Could you check a few things on this drawing? It's one solid part, dimensions in mm from its lowest x, y, z. A direction names the side the tool comes from. Round coordinates to 2 decimals unless told otherwise and drop trailing zeros. Write each loop counter-clockwise with the first axis right and the second up, starting at its lowest first coordinate (ties: lowest second). Pieces come first, ordered by that corner, then holes. Notation, with made-up numbers: (45, 86) -> (61, 86) arc R21 ccw to (61, 96) -> close; hole circle Ø3 at (16, 88.25). An arc over 180 degrees is marked (long way). Answer in a Markdown table with one row per item.
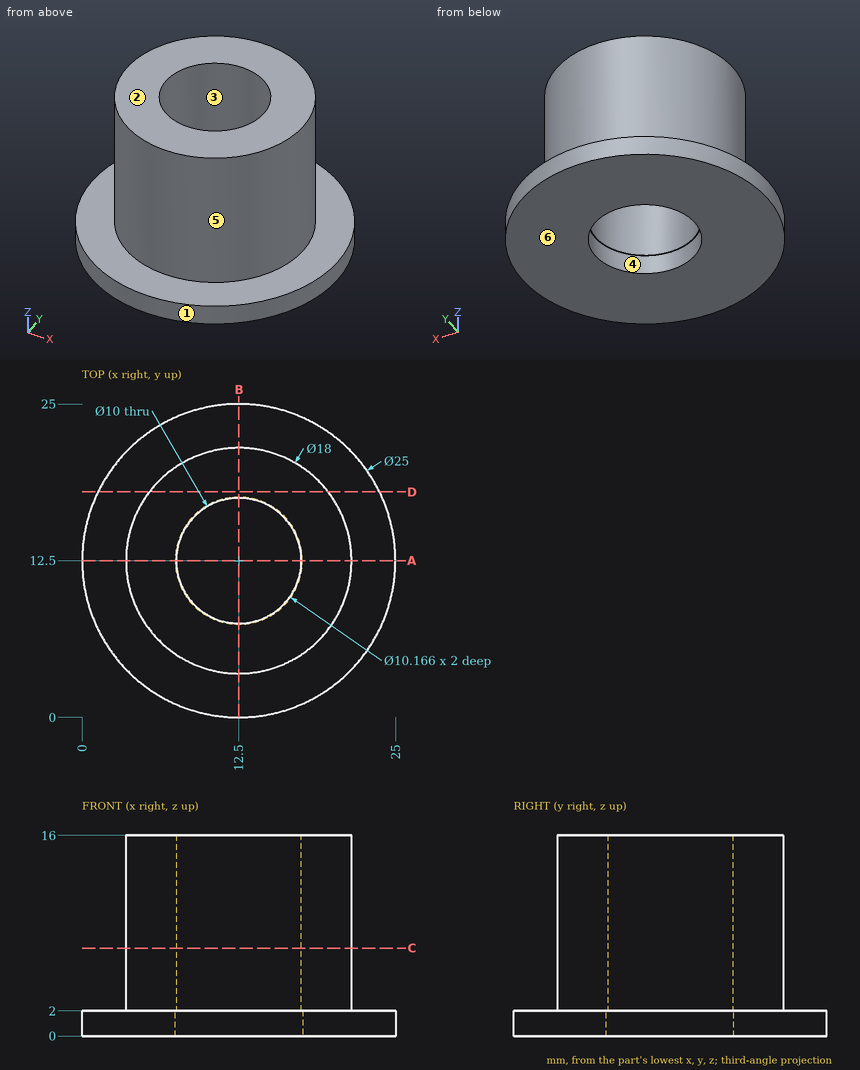
1) Imagine slicing it at A-A, the plane y = 12.5. Please give me the cut outline in (x, z).
Findings:
| item | result |
|---|---|
| outline | (0, 0) -> (7.42, 0) -> (7.42, 2) -> (7.5, 2) -> (7.5, 16) -> (3.5, 16) -> (3.5, 2) -> (0, 2) -> close; (17.5, 2) -> (17.58, 2) -> (17.58, 0) -> (25, 0) -> (25, 2) -> (21.5, 2) -> (21.5, 16) -> (17.5, 16) -> close |
2) Imagine slicing it at D-D, the plane y = 18. Please give me the cut outline in (x, z) (1 decimal).
Findings:
| item | result |
|---|---|
| outline | (1.3, 0) -> (23.7, 0) -> (23.7, 2) -> (19.6, 2) -> (19.6, 16) -> (5.4, 16) -> (5.4, 2) -> (1.3, 2) -> close |
3) Please list where these lines run through material, in increasing order: line 1 (Y direction, x = 12.5, z = 1.55); line 2 (X direction, y = 12.25, z = 14.5); line 3 (Y direction, x = 12.5, z = 5).
Findings:
| item | result |
|---|---|
| line 1 | y = 0 to 7.42, 17.58 to 25 |
| line 2 | x = 3.5 to 7.51, 17.49 to 21.5 |
| line 3 | y = 3.5 to 7.5, 17.5 to 21.5 |
4) Imagine slicing it at C-C, the plane z = 7. Please give me the cut outline in (x, y).
Findings:
| item | result |
|---|---|
| outline | circle Ø18 at (12.5, 12.5); hole circle Ø10 at (12.5, 12.5) |
5) For pin 1 (8 mm diameter, centred on x = 13, z = 7.5, fed in from +Y); pin 2 (1 mm diameter, centred on y = 10, z = 9.5, fed in from -X) (1 decimal); pin 3 (3 mm diameter, centred on x = 18.5, z = 10.5, fed in from -Y) (1 decimal), each with a flat end and sliding along its axis, tell me the tip position at first contact or that it passes through.
Findings:
| item | result |
|---|---|
| pin 1 | stops at y = 21.5 |
| pin 2 | stops at x = 3.7 |
| pin 3 | stops at y = 4.7 |
6) Thinking about a two-plate mould opening in Y: for the marked faces 1, 2 and 3, which applies, +Y half, -Y half, draft (parallel to the pull), parting line (faces both ways), or undercut?
Findings:
| item | result |
|---|---|
| face 1 | parting line |
| face 2 | draft |
| face 3 | undercut |
7) For the marked faces 4, 5 and 6, which set-ups out of +Z, -Z, +X, -X, +Y, -Y let a thin tool reach every point of the face, with its end or its side?
Findings:
| item | result |
|---|---|
| face 4 | -Z |
| face 5 | +Z |
| face 6 | -Z, +X, -X, +Y, -Y |
